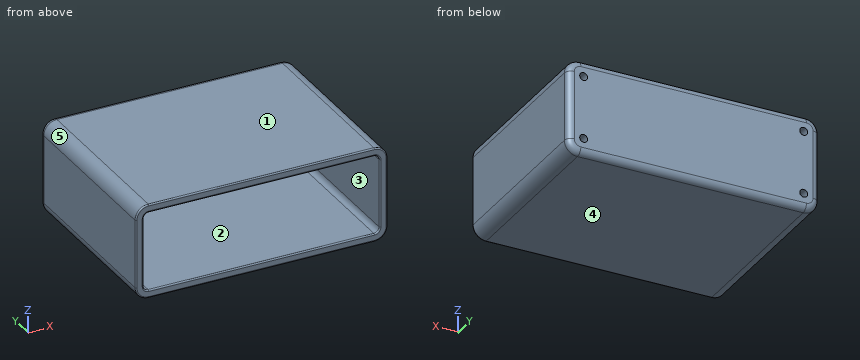
from build123d import *

# Parameters (mm, degrees)
BOSS_EXTRUDE1_DEPTH = 60
BOSS_EXTRUDE2_DEPTH = 10
FILLET1_R           = 2.5
FILLET2_R           = 0.5
SKETCH7_R           = 1.5
CUT_EXTRUDE1_DEPTH  = 10


with BuildPart() as part:
    # Sketch1 → Boss-Extrude1 (new body)
    with BuildSketch(Plane(origin=(0, 0, 0), x_dir=(1, 0, 0), z_dir=(0, 1, 0))):
        with BuildLine():
            Line((-43, 10.447552448), (43, 10.447552448))
            ThreePointArc((43, 10.447552448), (46.535533906, 8.983086353), (48, 5.447552448))
            Line((48, 5.447552448), (48, -20.552447552))
            ThreePointArc((48, -20.552447552), (46.535533906, -24.087981458), (43, -25.552447552))
            Line((43, -25.552447552), (-43, -25.552447552))
            ThreePointArc((-43, -25.552447552), (-46.535533906, -24.087981458), (-48, -20.552447552))
            Line((-48, -20.552447552), (-48, 5.447552448))
            ThreePointArc((-48, 5.447552448), (-46.535533906, 8.983086353), (-43, 10.447552448))
        make_face()
        with BuildLine():
            Line((-43, 7.447552448), (43, 7.447552448))
            ThreePointArc((43, 7.447552448), (44.414213562, 6.86176601), (45, 5.447552448))
            Line((45, 5.447552448), (45, -20.552447552))
            ThreePointArc((45, -20.552447552), (44.414213562, -21.966661115), (43, -22.552447552))
            Line((43, -22.552447552), (-43, -22.552447552))
            ThreePointArc((-43, -22.552447552), (-44.414213562, -21.966661115), (-45, -20.552447552))
            Line((-45, -20.552447552), (-45, 5.447552448))
            ThreePointArc((-45, 5.447552448), (-44.414213562, 6.86176601), (-43, 7.447552448))
        make_face(mode=Mode.SUBTRACT)
    extrude(amount=BOSS_EXTRUDE1_DEPTH)

    # Sketch2 → Boss-Extrude2 (add)
    with BuildSketch(Plane(origin=(0, 60, 0), x_dir=(1, 0, 0), z_dir=(0, 1, 0))):
        with BuildLine():
            Line((-43, -25.552447552), (43, -25.552447552))
            ThreePointArc((43, -25.552447552), (46.535533906, -24.087981458), (48, -20.552447552))
            Line((48, -20.552447552), (48, 5.447552448))
            ThreePointArc((48, 5.447552448), (46.535533906, 8.983086353), (43, 10.447552448))
            Line((43, 10.447552448), (-43, 10.447552448))
            ThreePointArc((-43, 10.447552448), (-46.535533906, 8.983086353), (-48, 5.447552448))
            Line((-48, 5.447552448), (-48, -20.552447552))
            ThreePointArc((-48, -20.552447552), (-46.535533906, -24.087981458), (-43, -25.552447552))
        make_face()
    extrude(amount=BOSS_EXTRUDE2_DEPTH)

    # Fillet1
    fillet1_edges = [part.edges().sort_by_distance(p)[0] for p in [
        (-46.535533906, 70, 24.087981458),
        (0, 70, 25.552447552),
        (46.535533906, 70, 24.087981458),
        (48, 70, 7.552447552),
        (46.535533906, 70, -8.983086353),
        (0, 70, -10.447552448),
        (-46.535533906, 70, -8.983086353),
        (-48, 70, 7.552447552),
    ]]
    fillet(fillet1_edges, radius=FILLET1_R)

    # Fillet2
    fillet2_edges = [part.edges().sort_by_distance(p)[0] for p in [
        (48, 0, 7.552447552),
        (46.535533906, 0, 24.087981458),
        (0, 0, 25.552447552),
        (-46.535533906, 0, 24.087981458),
        (-44.414213562, 0, -6.86176601),
        (-45, 0, 7.552447552),
        (-44.414213562, 0, 21.966661115),
        (0, 0, 22.552447552),
        (44.414213562, 0, 21.966661115),
        (45, 0, 7.552447552),
        (44.414213562, 0, -6.86176601),
        (0, 0, -7.447552448),
        (-48, 0, 7.552447552),
        (-46.535533906, 0, -8.983086353),
        (0, 0, -10.447552448),
        (46.535533906, 0, -8.983086353),
    ]]
    fillet(fillet2_edges, radius=FILLET2_R)

    # Sketch7 → Cut-Extrude1 (cut)
    with BuildSketch(Plane(origin=(0, 70, 0), x_dir=(1, 0, 0), z_dir=(0, 1, 0))):
        with Locations(Location((-41.939339828, 4.386892276, 0), (0, 0, 270))):
            Circle(SKETCH7_R)
        with Locations(Location((-41.939339828, -19.491787381, 0), (0, 0, 90))):
            Circle(SKETCH7_R)
        with Locations(Location((41.939339828, -19.491787381, 0), (0, 0, 270))):
            Circle(SKETCH7_R)
        with Locations(Location((41.939339828, 4.386892276, 0), (0, 0, 90))):
            Circle(SKETCH7_R)
    extrude(amount=-CUT_EXTRUDE1_DEPTH, mode=Mode.SUBTRACT)


solid = part.part
For this review, take the finished solid that the model builds, in its own axes (mm). Face numbers are marked on the shaded views. A direction names the side the tool comes from. Round coordinates to 2 decimals unless told otherwise and drop trailing zeros. Loops run counter-clockwise (first coordinate to the right, second up) from the corner with the lowest first, then second, coordinate; pieces in that order, holes last. Notation, with made-up numbers: (-25, 5) - (-7, 5) arc R11 ccw to (-7, 17) - close; hole circle Ø10 at (62.5, 69). An arc over 180 degrees is marked (long way). One line per item, written item: value. Start each with the question number.
Item 1: Take a section at A-A (y = 7). Give the boundary of the cut face in (x, z).
Item 2: For the marked faces 1 and 2, list the 3-axis set-ups (+Z, -Z, +X, -X, +Y, -Y) from which the entire face can be reached by the end or side of a thin tool; tool diameter is ignored.
Item 3: Take a section at B-B (z = 5). Give the boundary of the cut face in (x, y), plus the area to 3 significant figures.
Item 4: For L1, parallel to Z at x = 31, y = 11.5; L2, parallel to X at y = 47, z = 2; L3, parallel to Y at x = -38.5, z = 2, list the stretches that pass through material, from the lowest coordinate up.
Item 5: Take a section at C-C (x = 9). Give the boundary of the cut face in (y, z), plus the area to 3 significant figures.
Item 6: The part is to be moulded in two halves that separate along Z. For the marked faces 3, 4 and 5, say which applies: +Z half, -Z half, draft (parallel to the pull), parting line (faces both ways), or undercut.
Item 7: Clearance check with flat-ended pins moving along their axes: pin 1 Ø5 at (x, z) = (41.94, 19.49) entering from +Y; pin 2 Ø6 at (x, z) = (-31, 5) entering from -Y. State where each tip first meets the part, or that it passes through.
Answer below:
1. outline: (-48, -5.45) arc R5 ccw to (-43, -10.45) - (43, -10.45) arc R5 ccw to (48, -5.45) - (48, 20.55) arc R5 ccw to (43, 25.55) - (-43, 25.55) arc R5 ccw to (-48, 20.55) - close; hole (-45, -5.45) arc R2 ccw to (-43, -7.45) - (43, -7.45) arc R2 ccw to (45, -5.45) - (45, 20.55) arc R2 ccw to (43, 22.55) - (-43, 22.55) arc R2 ccw to (-45, 20.55) - close
2. face 1: +Z, +X, -X, +Y, -Y
2. face 2: -Y
3. outline: (-48, 0.5) arc R0.5 ccw to (-47.5, 0) - (-45.5, 0) arc R0.5 ccw to (-45, 0.5) - (-45, 60) - (45, 60) - (45, 0.5) arc R0.5 ccw to (45.5, 0) - (47.5, 0) arc R0.5 ccw to (48, 0.5) - (48, 67.5) arc R2.5 ccw to (45.5, 70) - (-45.5, 70) arc R2.5 ccw to (-48, 67.5) - close
3. area: 1,320 mm2
4. L1: z = -10.45 to -7.45, 22.55 to 25.55
4. L2: x = -48 to -45, 45 to 48
4. L3: y = 60 to 70
5. outline: (0, -9.95) arc R0.5 ccw to (0.5, -10.45) - (67.5, -10.45) arc R2.5 ccw to (70, -7.95) - (70, 23.05) arc R2.5 ccw to (67.5, 25.55) - (0.5, 25.55) arc R0.5 ccw to (0, 25.05) - (0, 23.05) arc R0.5 ccw to (0.5, 22.55) - (60, 22.55) - (60, -7.45) - (0.5, -7.45) arc R0.5 ccw to (0, -7.95) - close
5. area: 717 mm2
6. face 3: undercut
6. face 4: -Z half
6. face 5: +Z half
7. pin 1: stops at y = 70
7. pin 2: stops at y = 60
